from build123d import *

# Parameters (mm, degrees)
F0_W     = 16
F0_H     = 42
F0_R     = 1.75
F1_DEPTH = 2
F2_W     = 16
F2_H     = 5
F3_DEPTH = 24
F4_R     = 1.75
F5_DEPTH = 5


with BuildPart() as f1:
    # F0 (on Front) → F1 (new body)
    with BuildSketch(Plane.XZ):
        with Locations((8, 21)):
            Rectangle(F0_W, F0_H)
        with Locations((13.5, 3.5)):
            Circle(F0_R, mode=Mode.SUBTRACT)
        with Locations((13.5, 22.5)):
            Circle(F0_R, mode=Mode.SUBTRACT)
    extrude(amount=F1_DEPTH)

    # F2 (on face) → F3 (join)
    with BuildSketch(Plane(origin=(0, 0, 0), x_dir=(-1, 0, 0), z_dir=(0, 1, 0))):
        with Locations((-8, 44.5)):
            Rectangle(F2_W, F2_H)
    extrude(amount=-F3_DEPTH)

    # F4 (on face) → F5 (cut, through all)
    with BuildSketch(Plane(origin=(0, 0, 42), x_dir=(1, 0, 0), z_dir=(0, 0, -1))):
        with Locations((8, 14)):
            Circle(F4_R)
    extrude(amount=-F5_DEPTH, mode=Mode.SUBTRACT)


solid = f1.part
Can you work these out from the model? Positions are in its coordinate system, mm. A direction names the side the tool comes from. Give positions to 0.01 mm unless a question says otherwise; leave off trailing zeros. Order: outer loops, then holes, each group sorted by start corner. A loop starts at its lowest first (then second) coordinate and runs counter-clockwise, first axis right, second up. Notation, with made-up numbers: M 32.5,0.25 L 44.5,0.25 A29 cw 44.5,26.25 Z; hole C -1,-6 d2. An arc over 180 degrees is marked long. Use one line per item in the form item = value. Start each with the question number.
Item 1: If we section it at C-C (x = 13.5): Write out the boundary of the cut face in (y, z), then the cut area to 3 significant figures.
Item 2: If we section it at D-D (z = 22.5): Write out the boundary of the cut face in (x, y), then the cut area to 3 significant figures.
Item 3: If we section it at B-B (y = -14): Write out the boundary of the cut face in (x, z).
Item 4: If we section it at A-A (x = 8): Write out the boundary of the cut face in (y, z).
Item 5: If I drill on line 1 along Z through (x, y) = (13.5, -1.1); line 2 along X through (y, z) = (-14, 44.3); line 3 along Y through (x, z) = (2, 30.5), over which ranges is the centre line in solid material (lowest first)?
Item 6: For faces 4 (the flat face through (8, -12, 47)), 5 (the flat face through (10, -13, 42)), which set-ups out of +Z, -Z, +X, -X, +Y, -Y let a thin tool reach every point of the face, with its end or its side?
Item 7: Will these pins go through, and if not, where does the flat tip stop? pin 1 Ø6 at (x, y) = (14, -11.5) entering from -Z; pin 2 Ø5 at (x, z) = (4.5, 19.5) entering from -Y; pin 3 Ø6 at (y, z) = (-21, 37) entering from +X.
Item 8: We'd pull the mould along Y, two halves only. Please class faces 1 (the flat face through (8, -2, 21)), 2 (the flat face through (8, 0, 24)), 3 (the cylindrical face through (7.772, -15.735, 44.465)): +Y half, -Y half, draft (parallel to the pull), parting line (faces both ways), or undercut.
Outcome:
q1.outline = M -24,42 L -2,42 L -2,24.25 L 0,24.25 L 0,47 L -24,47 Z; M -2,0 L 0,0 L 0,1.75 L -2,1.75 Z; M -2,5.25 L 0,5.25 L 0,20.75 L -2,20.75 Z
q1.area = 190 mm2
q2.outline = M 0,-2 L 11.75,-2 L 11.75,0 L 0,0 Z; M 15.25,-2 L 16,-2 L 16,0 L 15.25,0 Z
q2.area = 25.0 mm2
q3.outline = M 0,42 L 6.25,42 L 6.25,47 L 0,47 Z; M 9.75,42 L 16,42 L 16,47 L 9.75,47 Z
q4.outline = M -24,42 L -15.75,42 L -15.75,47 L -24,47 Z; M -12.25,42 L -2,42 L -2,0 L 0,0 L 0,47 L -12.25,47 Z
q5.line_1 = 0 to 1.75, 5.25 to 20.75, 24.25 to 47
q5.line_2 = 0 to 6.25, 9.75 to 16
q5.line_3 = -2 to 0
q6.face_4 = +Z, +X, -X, +Y, -Y
q6.face_5 = -Z, +X, -X, -Y
q7.pin_1 = 42
q7.pin_2 = -2
q7.pin_3 = through
q8.face_1 = -Y half
q8.face_2 = +Y half
q8.face_3 = undercut
